Build history of the part. All positions in model axes, mm. A direction names the side the tool comes from. Coordinates: 2 decimals unless noted, no trailing zeros. Write each loop counter-clockwise with the first axis right and the second up, starting at its lowest first coordinate (ties: lowest second). Pieces come first, ordered by that corner, then holes.
```python
from build123d import *

# Parameters (mm, degrees)
SKETCH1_R           = 13
SKETCH1_R_2         = 4.25
BOSS_EXTRUDE1_DEPTH = 1.25


with BuildPart() as part:
    # Sketch1 → Boss-Extrude1 (new body, symmetric)
    with BuildSketch(Plane(origin=(0, 0, 0), x_dir=(1, 0, 0), z_dir=(0, 1, 0))):
        with BuildLine():
            Line((-21.223783798, -59.5), (23.776216202, -59.5))
            Line((23.776216202, -59.5), (19.918131719, -48.9))
            Line((19.918131719, -48.9), (44.905089026, -32.046084487))
            Line((44.905089026, -32.046084487), (13.660617354, 10.13521746))
            ThreePointArc((13.660617354, 10.13521746), (-0.749839352, 17), (-14.499227131, 8.891927633))
            Line((-14.499227131, 8.891927633), (-46.094910974, -42.724212896))
            Line((-46.094910974, -42.724212896), (-21.223783798, -59.5))
        make_face()
        Circle(SKETCH1_R, mode=Mode.SUBTRACT)
        with Locations((22.405089026, -29.5)):
            Circle(SKETCH1_R_2, mode=Mode.SUBTRACT)
    extrude(amount=BOSS_EXTRUDE1_DEPTH, both=True)


solid = part.part
```
1. Flat gauge pins, fed straight in: pin 1 (1 mm diameter, centred on x = -20, y = 0, fed in from -Z); pin 2 (15.5 mm diameter, centred on x = 0, z = 0, fed in from +Y). Where does each tip first touch, or does it go through?
Computed values:
pin 1: stops at z = -0.72
pin 2: passes through
2. Mould opens along X. For faces 1 (the face through (-0.52, 0.02, -17.01)), 2 (the face through (-10.316, -0.018, 7.91)), 3 (the face through (1, 0, 59.5)) say: +X half, -X half, draft (parallel to the pull), parting line (faces both ways), or undercut.
Computed values:
face 1: parting line
face 2: undercut
face 3: draft
3. Probe line 1 along Z through (x, y) = (0, 0.05); line 2 along Z through (x, y) = (25, 0.8); line 3 along X through (y, z) = (-0.45, 2). List the from-to ranges inside material, lowest first.
Computed values:
line 1: z = -17.02 to -13, 13 to 59.5
line 2: z = 5.17 to 26.13, 32.87 to 45.47
line 3: x = -21.17 to -12.85, 12.85 to 22.65
4. Saw through at A-A on x = 0. List the corners of the cut face in (y, z).
Computed values:
outline: (-1.25, -17.02) - (1.25, -17.02) - (1.25, -13) - (-1.25, -13) - close; (-1.25, 13) - (1.25, 13) - (1.25, 59.5) - (-1.25, 59.5) - close
5. Saw through at C-C on y = -0.4. List the corners of the cut face in (x, z), plus the area to 3 significant figures.
Computed values:
outline: (-46.09, 42.72) - (-14.5, -8.89) arc R17 ccw to (13.66, -10.14) - (44.91, 32.05) - (19.92, 48.9) - (23.78, 59.5) - (-21.22, 59.5) - close; hole circle Ø26 at (0, 0); hole circle Ø8.5 at (22.41, 29.5)
area: 3,700 mm2
6. 3-axis set-ups, long thin cutter, end or side, ignore diameter. For faces 4 (the face through (21.874, 0.018, 54.274)), 5 (the face through (-33.833, 0.018, 50.995)): which of +Z, -Z, +X, -X, +Y, -Y reach the whole face in a straight line?
Computed values:
face 4: +X, +Y, -Y
face 5: +Z, -X, +Y, -Y
7. Saw through at B-B on z = 0. List the corners of the cut face in (x, y).
Computed values:
outline: (-19.94, -1.25) - (-13, -1.25) - (-13, 1.25) - (-19.94, 1.25) - close; (13, -1.25) - (21.17, -1.25) - (21.17, 1.25) - (13, 1.25) - close
8. Saw through at D-D on z = 21. List the corners of the cut face in (x, y).
Computed values:
outline: (-32.8, -1.25) - (36.72, -1.25) - (36.72, 1.25) - (-32.8, 1.25) - close
